Here's how the part is built. I have some questions about the finished solid (model axes, mm). Give positions to 0.01 mm unless a question says otherwise; leave off trailing zeros. One line per item, written item: value. Start each with the question number.
1) Please list where this line runs through material, in increasing order: L1, parallel to Z at x = -2.75, y = -0.5. Write a range as [from, to].
2) We'd pull the mould along Y, two halves only. Please class faces 1 (the flat face through (-9.532, -2, 7)), 2 (the flat face through (-2, -2, 0.5)), 3 (the flat face through (-2, -9.555, 7)): +Y half, -Y half, draft (parallel to the pull), parting line (faces both ways), or undercut.
3) I'm going to push a flat-ended pin straight in: P1, Ø3.5, axis at x = -2.03, y = -2.06, coming from the -Z side. Where does the tip first touch, or does it pass through?
from build123d import *

# Parameters (mm, degrees)
F0_W     = 15
F0_H     = 15
F1_DEPTH = 15
F2_R     = 1.5
F3_DEPTH = 0.5
F4_R     = 0.5
F5_R     = 0.24999


# Not quite as in the source:
# - a fillet or chamfer is up to 0.001 mm smaller than in the source, because OpenCascade refuses the exact size
# - a feature names something its author has since deleted; it is built from what else it names


with BuildPart() as f1:
    # F0 (on Top) → F1 (new body)
    with BuildSketch(Plane.XY):
        with Locations((-2.0319856703, -2.0552466768)):
            Rectangle(F0_W, F0_H)
    extrude(amount=F1_DEPTH)

    # F2 (on face) → F3 (cut)
    with BuildSketch(Plane(origin=(0, 0, 0), x_dir=(1, 0, 0), z_dir=(0, 0, -1))):
        with Locations((-2.0319856703, 2.0552456845)):
            Circle(F2_R)
    extrude(amount=-F3_DEPTH, mode=Mode.SUBTRACT)

    # F4
    f4_edges = [f1.edges().sort_by_distance(p)[0] for p in [
        (5.468014, 5.444753, 7.5),
        (-2.031986, 5.444753, 0),
        (-2.031986, 5.444753, 15),
        (-9.531986, 5.444753, 7.5),
        (5.468014, -2.055247, 0),
        (5.468014, -2.055247, 15),
        (5.468014, -9.555247, 7.5),
        (-9.531986, -2.055247, 0),
        (-2.031986, -9.555247, 0),
        (-9.531986, -2.055247, 15),
        (-9.531986, -9.555247, 7.5),
        (-2.031986, -9.555247, 15),
    ]]
    fillet(f4_edges, radius=F4_R)

    # F5 (radius 0.25 in the source; OpenCascade refuses exactly that, so slightly less here)
    f5_edges = [f1.edges().sort_by_distance(p)[0] for p in [
        (-3.531986, -2.055246, 0.5),
        (-3.531986, -2.055246, 0),
    ]]
    fillet(f5_edges, radius=F5_R)


solid = f1.part
Numbers:
1. L1: [0, 15]
2. face 1: draft
2. face 2: undercut
2. face 3: -Y half
3. P1: z = 0
